Here's how the part is built. I have some questions about the finished solid (model axes, mm). Face numbers are marked on the shaded views. Coordinates: 2 decimals unless noted, no trailing zeros. Write each loop counter-clockwise with the first axis right and the second up, starting at its lowest first coordinate (ties: lowest second). Pieces come first, ordered by that corner, then holes. Notation, with made-up numbers: (67.5, 66) -> (77.5, 66) arc R24 cw to (77.5, 76) -> close; hole circle Ø8 at (18, 82.5). An arc over 180 degrees is marked (long way). Put each result on its own line as item: value.
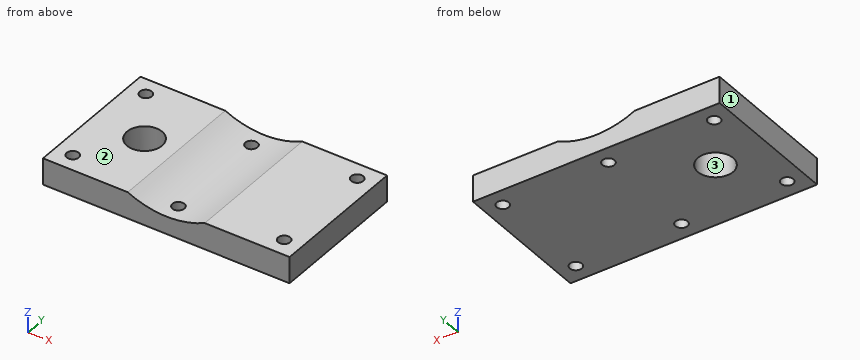
```python
from build123d import *

# Parameters (mm, degrees)
F0_W     = 44.45
F0_H     = 25.4
F1_DEPTH = 4.7752
F2_R     = 1.0922
F2_R_2   = 3.175
F3_DEPTH = 4.7762
F4_R     = 15.875
F5_DEPTH = 25.401


with BuildPart() as f1:
    # F0 (on Top) → F1 (new body)
    with BuildSketch(Plane.XY):
        Rectangle(F0_W, F0_H)
    extrude(amount=F1_DEPTH)

    # F2 (on face) → F3 (cut, through all)
    with BuildSketch(Plane.XY.offset(4.7752)):
        with Locations((-19.05, 9.525)):
            Circle(F2_R)
        with Locations((19.05, 9.525)):
            Circle(F2_R)
        with Locations((19.05, -9.525)):
            Circle(F2_R)
        with Locations((-19.05, -9.525)):
            Circle(F2_R)
        with Locations((-12.7, 0)):
            Circle(F2_R_2)
        with Locations((0, 9.525)):
            Circle(F2_R)
        with Locations((0, -9.525)):
            Circle(F2_R)
    extrude(amount=-F3_DEPTH, mode=Mode.SUBTRACT)

    # F4 (on face) → F5 (cut, through all)
    with BuildSketch(Plane.XZ.offset(12.7)):
        with Locations((0, 19.05)):
            Circle(F4_R)
    extrude(amount=-F5_DEPTH, mode=Mode.SUBTRACT)


solid = f1.part
```
Item 1: Imagine slicing it at C-C on y = 0. Write out the boundary of the cut face in (x, z) (3 decimals), then the cut area to 3 significant figures.
Output:
outline: (-22.225, 0) -> (-15.875, 0) -> (-15.875, 4.775) -> (-22.225, 4.775) -> close; (-9.525, 0) -> (22.225, 0) -> (22.225, 4.775) -> (6.946, 4.775) arc R15.875 cw to (-6.946, 4.775) -> (-9.525, 4.775) -> close
area: 167 mm²
Item 2: If we mould it in two halves opening along X, with no side actions, what happens to the marked faces 1, 2 and 3? For each: released by +X, released by -X, zero draft, split by the parting line, or undercut.
Output:
face 1: released by -X
face 2: zero draft
face 3: undercut
Item 3: For P1, Ø1.3, axis at x = -19.05, y = -9.525, coming from the +Z side; P2, Ø2.5, axis at x = 0, y = 9.525, coming from the +Z side, each with a flat end and sliding along its axis, tell me the tip position at first contact or that it passes through.
Output:
P1: passes through
P2: stops at z = 3.22
Item 4: Imagine slicing it at D-D on x = -19.05. Write out the boundary of the cut face in (y, z).
Output:
outline: (-12.7, 0) -> (-10.62, 0) -> (-10.62, 4.78) -> (-12.7, 4.78) -> close; (-8.43, 0) -> (8.43, 0) -> (8.43, 4.78) -> (-8.43, 4.78) -> close; (10.62, 0) -> (12.7, 0) -> (12.7, 4.78) -> (10.62, 4.78) -> close
Item 5: Please list where these lines run through material, in increasing order: line 1 along Y through (x, z) = (-19, 3.3); line 2 along X through (y, z) = (-10, 0.65) (1 decimal); line 3 along Y through (x, z) = (-12.7, 1.85) (3 decimals). Write a range as from..to.
Output:
line 1: y = -12.7..-10.62, -8.43..8.43, 10.62..12.7
line 2: x = -22.2..-20, -18.1..-1, 1..18.1, 20..22.2
line 3: y = -12.7..-3.175, 3.175..12.7
Item 6: Imagine slicing it at B-B on z = 4.1. Write out the boundary of the cut face in (x, y) (3 decimals), then the cut area to 3 significant figures.
Output:
outline: (-22.225, -12.7) -> (-5.34, -12.7) -> (-5.34, 12.7) -> (-22.225, 12.7) -> close; (5.34, -12.7) -> (22.225, -12.7) -> (22.225, 12.7) -> (5.34, 12.7) -> close; hole circle Ø2.184 at (-19.05, -9.525); hole circle Ø2.184 at (-19.05, 9.525); hole circle Ø6.35 at (-12.7, 0); hole circle Ø2.184 at (19.05, -9.525); hole circle Ø2.184 at (19.05, 9.525)
area: 811 mm²
Item 7: Imagine slicing it at A-A on x = -12.7. Write out the boundary of the cut face in (y, z) (3 decimals), then the cut area to 3 significant figures.
Output:
outline: (-12.7, 0) -> (-3.175, 0) -> (-3.175, 4.775) -> (-12.7, 4.775) -> close; (3.175, 0) -> (12.7, 0) -> (12.7, 4.775) -> (3.175, 4.775) -> close
area: 91.0 mm²
